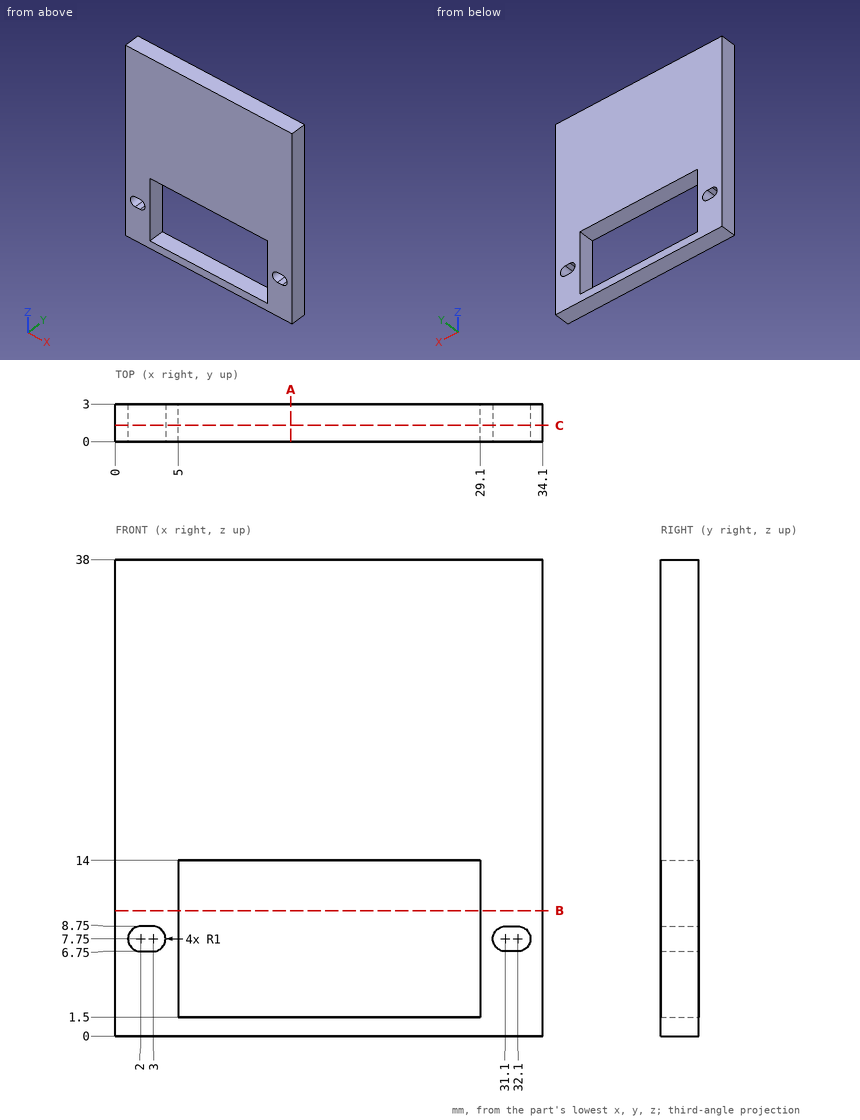
Design review of the part shown in the three views and the two pictorial views. Dimensions are in mm from the part's minimum x, y and z. Round coordinates to 2 decimals unless told otherwise and drop trailing zeros. Write each loop counter-clockwise with the first axis right and the second up, starting at its lowest first coordinate (ties: lowest second). Pieces come first, ordered by that corner, then holes. Notation, with made-up numbers: (51.25, -23.75) - (92.25, -23.75) arc R13 cw to (92.25, -5.75) - close; hole circle Ø1 at (20.25, 73.25). An arc over 180 degrees is marked (long way). Return JSON: item names as keys, results as strings. Group by question number.
Item 1: For probe 1 along X at (y, z) = (2.05, 6); probe 2 along Z at (x, y) = (6, 1.9); probe 3 along Z at (x, y) = (32, 1.3), list the stretches that pass through material, from the lowest coordinate up. Write a range as [from, to].
Item 2: We need section C-C on y = 1.3. Write out the cut boundary in (x, z).
Item 3: We need section B-B on z = 10. Write out the cut boundary in (x, y), and give its area (3 significant figures).
Item 4: We need section A-A on x = 14. Write out the cut boundary in (y, z), and give its area (3 significant figures).
Model answer:
{
 "1": {"probe 1": "x = [0, 5], [29.1, 34.1]", "probe 2": "z = [0, 1.5], [14, 38]", "probe 3": "z = [0, 6.75], [8.75, 38]"},
 "2": {"outline": "(0, 0) - (34.1, 0) - (34.1, 38) - (0, 38) - close; hole (2, 6.75) - (3, 6.75) arc R1 ccw to (3, 8.75) - (2, 8.75) arc R1 ccw to start; hole (5, 1.5) - (29.1, 1.5) - (29.1, 14) - (5, 14) - close; hole (31.1, 6.75) - (32.1, 6.75) arc R1 ccw to (32.1, 8.75) - (31.1, 8.75) arc R1 ccw to start"},
 "3": {"outline": "(0, 0) - (5, 0) - (5, 3) - (0, 3) - close; (29.1, 0) - (34.1, 0) - (34.1, 3) - (29.1, 3) - close", "area": "30.0 mm²"},
 "4": {"outline": "(0, 0) - (3, 0) - (3, 1.5) - (0, 1.5) - close; (0, 14) - (3, 14) - (3, 38) - (0, 38) - close", "area": "76.5 mm²"}
}
